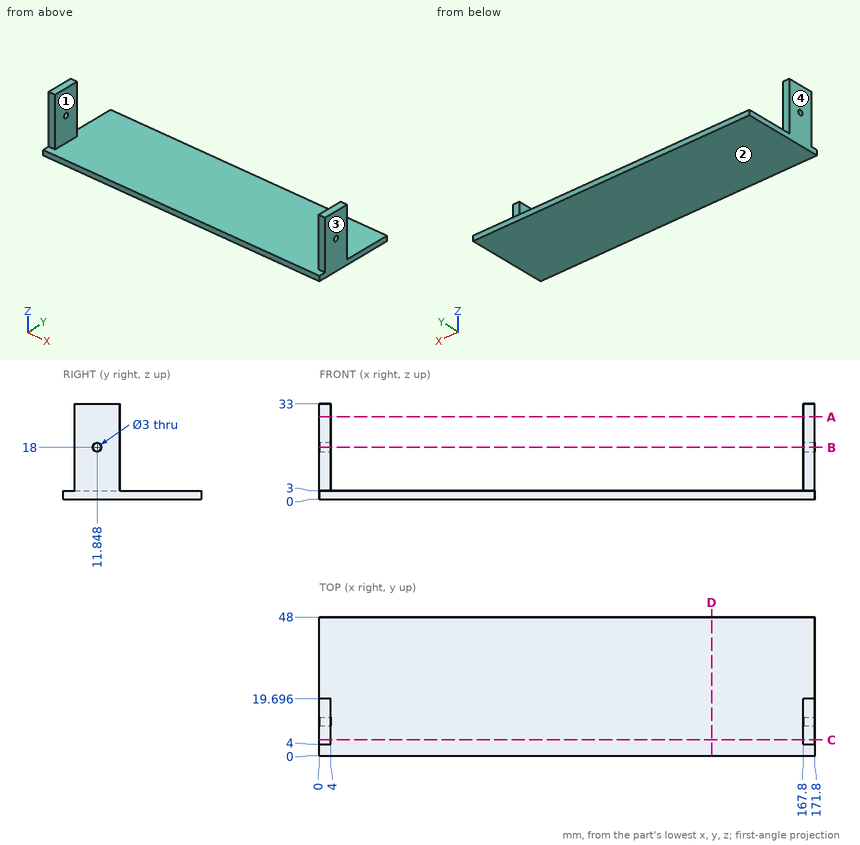
Drawing for the job (mm, zero at the part's lowest x, y, z). Coordinates: 2 decimals unless noted, no trailing zeros. Write each loop counter-clockwise with the first axis right and the second up, starting at its lowest first coordinate (ties: lowest second). Pieces come first, ordered by that corner, then holes. Notation, with made-up numbers: (20.5, 86.5) -> (66.5, 86.5) arc R21 ccw to (66.5, 115.5) -> close; hole circle Ø7 at (83.25, -27.75). An arc over 180 degrees is marked (long way). One line per item, written item: value. Start each with the question number.
1) Slice it at B-B on z = 18. Write the cut outline in (x, y), then the cut area to 3 significant figures.
2) Pull direction X, two halves, no side cores. Call the marked faces 1, 2, 3 and 4: +X half, -X half, draft (parallel to the pull), parting line (faces both ways), or undercut.
3) Slice it at A-A on z = 28.5. Write the cut outline in (x, y).
4) Flat gauge pins, fed straight in: pin 1 Ø3 at (x, z) = (2.5, 25) entering from +Y; pin 2 Ø3 at (x, z) = (169, 20) entering from -Y; pin 3 Ø1.8 at (y, z) = (11.85, 18) entering from +X; pin 4 Ø6 at (x, y) = (128.5, 28.5) entering from +Z. Where does each tip first touch, or does it go through?
5) Slice it at D-D on x = 136. Write the cut outline in (y, z).
6) Probe probe 1 along X at (y, z) = (13.5, 18); probe 2 along Z at (x, y) = (45, 38). List the from-to ranges inside material, lowest first.
7) Slice it at C-C on y = 5.5. Write the cut outline in (x, z).
Answers follow:
1. outline: (0, 4) -> (4, 4) -> (4, 10.35) -> (0, 10.35) -> close; (0, 13.35) -> (4, 13.35) -> (4, 19.7) -> (0, 19.7) -> close; (167.8, 4) -> (171.8, 4) -> (171.8, 10.35) -> (167.8, 10.35) -> close; (167.8, 13.35) -> (171.8, 13.35) -> (171.8, 19.7) -> (167.8, 19.7) -> close
1. area: 102 mm2
2. face 1: undercut
2. face 2: draft
2. face 3: +X half
2. face 4: -X half
3. outline: (0, 4) -> (4, 4) -> (4, 19.7) -> (0, 19.7) -> close; (167.8, 4) -> (171.8, 4) -> (171.8, 19.7) -> (167.8, 19.7) -> close
4. pin 1: y = 19.7
4. pin 2: y = 4
4. pin 3: through
4. pin 4: z = 3
5. outline: (0, 0) -> (48, 0) -> (48, 3) -> (0, 3) -> close
6. probe 1: 0 to 4, 167.8 to 171.8
6. probe 2: 0 to 3
7. outline: (0, 0) -> (171.8, 0) -> (171.8, 33) -> (167.8, 33) -> (167.8, 3) -> (4, 3) -> (4, 33) -> (0, 33) -> close
